from build123d import *

# Parameters (mm, degrees)
SKETCH_1_R              = 2
EXTRUDE_1_DEPTH         = 10
CUT_EXTRUDE_START       = -16
CUT_EXTRUDE_1_OUTLINE_R = 2
CUT_EXTRUDE_1_DEPTH     = 16


# Read off the part's stored shape, not the designer's step: 切除-拉伸1
with BuildPart() as part:
    # 草图1 → 凸台-拉伸1 (new body)
    with BuildSketch(Plane(origin=(0, 0, 0), x_dir=(1, 0, 0), z_dir=(0, 1, 0))):
        Polygon((-14.375, 0), (-2.375, 0), (-2.375, 4), (5.625, 4), (5.625, 0), (17.625, 0), (17.625, 16), (-14.375, 16), align=None)
        with Locations(Location((-6.230357992, 7.870924175, 0), (0, 0, 270))):
            Circle(SKETCH_1_R, mode=Mode.SUBTRACT)
        with Locations(Location((9.480357992, 7.870924175, 0), (0, 0, 90))):
            Circle(SKETCH_1_R, mode=Mode.SUBTRACT)
    extrude(amount=EXTRUDE_1_DEPTH)

    # 切除-拉伸1 outline → 切除-拉伸1 (cut)
    with BuildSketch(Plane.XY.offset(CUT_EXTRUDE_START)):
        with Locations((14.884036252, 5)):
            Circle(CUT_EXTRUDE_1_OUTLINE_R)
        with Locations((-11.634036252, 5)):
            Circle(CUT_EXTRUDE_1_OUTLINE_R)
    extrude(amount=CUT_EXTRUDE_1_DEPTH, mode=Mode.SUBTRACT)


solid = part.part
Could you check a few things on this model? Use its own coordinates, in mm. A direction names the side the tool comes from. Give positions to 0.01 mm unless a question says otherwise; leave off trailing zeros. Loops run counter-clockwise (first coordinate to the right, second up) from the corner with the lowest first, then second, coordinate; pieces in that order, holes last. Notation, with made-up numbers: M 49,-1 L 83,-1 A22 ccw 83,19 Z; hole C 66,46.25 d8. An arc over 180 degrees is marked long. Answer as a JSON object with one key per item and string values.
Q1. Suppose I cut it at C-C, the plane x = 15.5. List the corners of the cut face in (y, z) for me, plus the area to 3 significant figures.
Values found:
{"outline": "M 0,-16 L 3.1,-16 L 3.1,0 L 0,0 Z; M 6.9,-16 L 10,-16 L 10,0 L 6.9,0 Z", "area": "99.1 mm²"}
Q2. Suppose I cut it at B-B, the plane y = 5.75. List the corners of the cut face in (x, z) for me (3 decimals).
Values found:
{"outline": "M -14.375,-16 L -13.488,-16 L -13.488,0 L -14.375,0 Z; M -9.78,-16 L 13.03,-16 L 13.03,0 L 5.625,0 L 5.625,-4 L -2.375,-4 L -2.375,0 L -9.78,0 Z; M 16.738,-16 L 17.625,-16 L 17.625,0 L 16.738,0 Z; hole C -6.23,-7.871 d4; hole C 9.48,-7.871 d4"}
Q3. Suppose I cut it at A-A, the plane z = -8.75. List the corners of the cut face in (x, y) for me (3 decimals).
Values found:
{"outline": "M -14.375,0 L -8.027,0 L -8.027,10 L -14.375,10 Z; M -4.434,0 L 7.684,0 L 7.684,10 L -4.434,10 Z; M 11.277,0 L 17.625,0 L 17.625,10 L 11.277,10 Z; hole C -11.634,5 d4; hole C 14.884,5 d4"}
Q4. If we mould it in two halves opening along Z, with no side actions, what happens to faces 3 (the flat face through (-8, 5, 0)), 4 (the flat face through (1, 10, -8)), 5 (the cylindrical face through (-5.63, 4.93, -5.963))? For each: pulls with the +Z half, pulls with the -Z half, needs draft (parallel to the pull), parting line crosses it, or undercut.
Values found:
{"face 3": "pulls with the +Z half", "face 4": "needs draft", "face 5": "undercut"}
Q5. Suppose I cut it at D-D, the plane y = 7.75. List the corners of the cut face in (x, z) for me (3 decimals), plus the area to 3 significant figures.
Values found:
{"outline": "M -14.375,-16 L 17.625,-16 L 17.625,0 L 5.625,0 L 5.625,-4 L -2.375,-4 L -2.375,0 L -14.375,0 Z; hole C -6.23,-7.871 d4; hole C 9.48,-7.871 d4", "area": "455 mm²"}
Q6. If I drill on probe 1 along X at (y, z) = (1.5, -7.75) (3 decimals); probe 2 along X at (y, z) = (3.5, -10) (3 decimals); probe 3 along X at (y, z) = (8.5, -3) (3 decimals), over which ranges is the centre line in solid material (lowest first)? Write a range as [from, to].
Values found:
{"probe 1": "x = [-14.375, -8.227], [-4.234, 7.484], [11.477, 17.625]", "probe 2": "x = [-14.375, -12.957], [-10.311, 13.561], [16.207, 17.625]", "probe 3": "x = [-14.375, -2.375], [5.625, 17.625]"}
Q7. For faces 1 (the flat face through (2, 5, -4)), 2 (the cylindrical face through (-13.632, 5.088, -8.112)), which set-ups out of +Z, -Z, +X, -X, +Y, -Y let a thin tool reach every point of the face, with its end or its side?
Values found:
{"face 1": "+Z, +Y, -Y", "face 2": "+Z, -Z"}
Q8. For P1, Ø3, axis at x = -6.23, z = -7.87, coming from the -Y side, with a flat end and sliding along its axis, tell me the tip position at first contact or that it passes through.
Values found:
{"P1": "passes through"}
